Can you work these out from the drawing? Everything is in mm from the part's minimum corner. A direction names the side the tool comes from. Give positions to 0.01 mm unless a question says otherwise; leave off trailing zeros. Order: outer loops, then holes, each group sorted by start corner. A loop starts at its lowest first (then second) coordinate and runs counter-clockwise, first axis right, second up. Notation, with made-up numbers: (3, 22.25) -> (59, 22.25) arc R24 ccw to (59, 60.25) -> close; hole circle Ø2 at (-30, 80.25). An arc over 180 degrees is marked (long way). One line per item, written item: value.
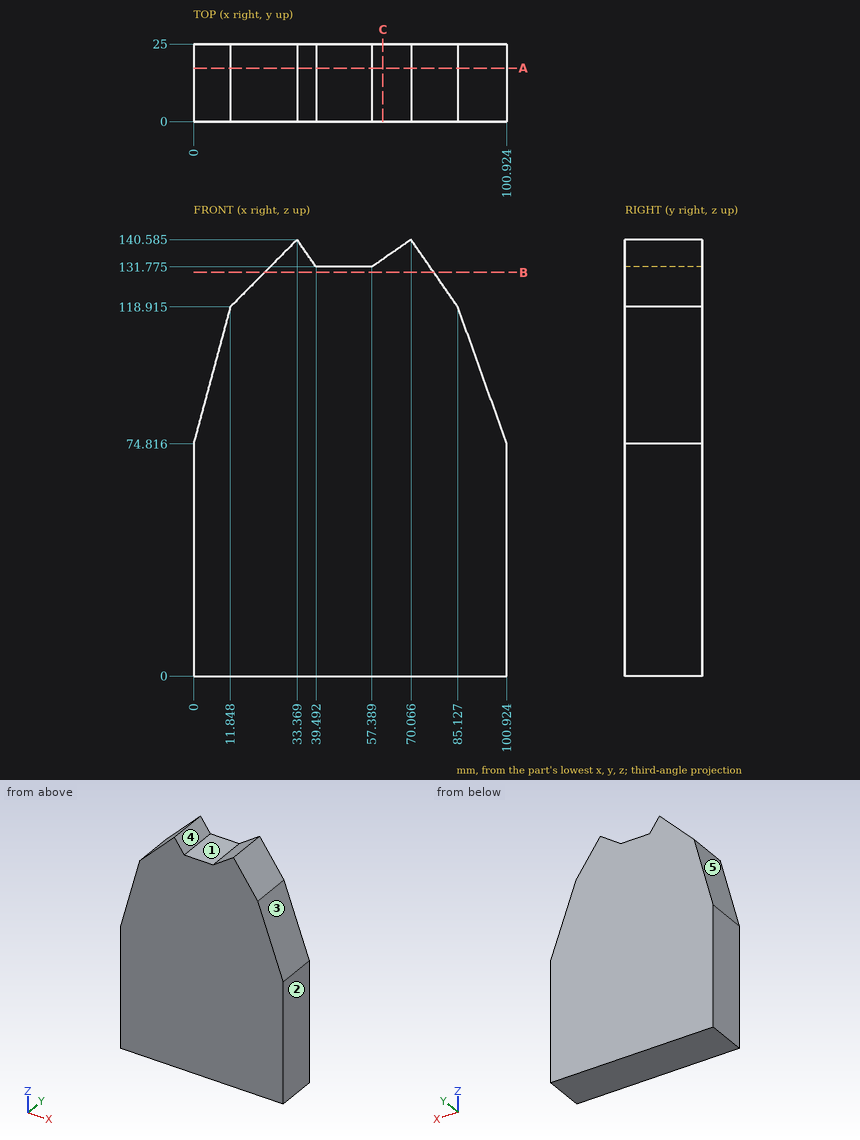
1) If I drill on line 1 along Z through (x, y) = (45.5, 9.75) (1 decimal); line 2 along Z through (x, y) = (69, 5.75) (1 decimal); line 3 along X through (y, z) = (16.5, 117) (1 decimal), over which ranges is the centre line in solid material (lowest first)?
Answer below:
line 1: z = 0 to 131.8
line 2: z = 0 to 139.8
line 3: x = 11.3 to 85.8
2) We'd pull the mould along X, two halves only. Please class the marked faces 3, 4 and 5: +X half, -X half, draft (parallel to the pull), parting line (faces both ways), or undercut.
Answer below:
face 3: +X half
face 4: undercut
face 5: -X half
3) Suppose I cut it at B-B, the plane z = 130. Write out the boundary of the cut face in (x, y), then the cut area to 3 significant figures.
Answer below:
outline: (22.86, 0) -> (77.42, 0) -> (77.42, 25) -> (22.86, 25) -> close
area: 1,360 mm2
4) Suppose I cut it at C-C, the plane x = 61. Write out the boundary of the cut face in (y, z) (1 decimal), then the cut area to 3 significant figures.
Answer below:
outline: (0, 0) -> (25, 0) -> (25, 134.3) -> (0, 134.3) -> close
area: 3,360 mm2
5) For the marked faces 1 and 2, which set-ups out of +Z, -Z, +X, -X, +Y, -Y let a thin tool reach every point of the face, with its end or its side?
Answer below:
face 1: +Z, +Y, -Y
face 2: +Z, -Z, +X, +Y, -Y
6) For P1, Ø4, axis at x = 67.5, y = 5, coming from the +Z side; P2, Ø1.5, axis at y = 14.5, z = 87.5, coming from the -X side; P3, Ø2, axis at y = 5.5, z = 95, coming from the -X side, each with a flat end and sliding along its axis, tell me the tip position at first contact or that it passes through.
Answer below:
P1: stops at z = 140.19
P2: stops at x = 3.21
P3: stops at x = 5.15
7) Suppose I cut it at A-A, the plane y = 17.25. Write out the boundary of the cut face in (x, z) (1 decimal).
Answer below:
outline: (0, 0) -> (100.9, 0) -> (100.9, 74.8) -> (85.1, 118.9) -> (70.1, 140.6) -> (57.4, 131.8) -> (39.5, 131.8) -> (33.4, 140.6) -> (11.8, 118.9) -> (0, 74.8) -> close
